```python
from build123d import *

# Parameters (mm, degrees)
SKETCH1_W           = 90
SKETCH1_H           = 34
BOSS_EXTRUDE1_DEPTH = 23.5
SKETCH2_R           = 1.8
BOSS_EXTRUDE4_DEPTH = 10
FILLET1_R           = 3


with BuildPart() as part:
    # Sketch1 → Boss-Extrude1 (new body)
    with BuildSketch(Plane(origin=(0, 0, 0), x_dir=(1, 0, 0), z_dir=(0, 1, 0))):
        with Locations((2.348643006, -1.686847599)):
            Rectangle(SKETCH1_W, SKETCH1_H)
    extrude(amount=BOSS_EXTRUDE1_DEPTH)

    # Sketch2 → Boss-Extrude4 (add)
    with BuildSketch(Plane(origin=(47.348643006, 0, 0), x_dir=(0, 0, -1), z_dir=(1, 0, 0))):
        with Locations(Location((-16.886847599, 13.57, 0), (0, 0, 180))):
            Circle(SKETCH2_R)
        with Locations(Location((-16.886847599, 9.93, 0), (0, 0, 180))):
            Circle(SKETCH2_R)
    extrude(amount=BOSS_EXTRUDE4_DEPTH)

    # Fillet1
    # the kernel refuses this fillet: 3 mm, written as the material it takes off along each edge
    with BuildSketch(Plane(origin=(44.348643006, 20.5, -12.313152401), x_dir=(1, 0, 0), z_dir=(0, 0, -1))) as fillet1_piece_1_section:
        Polygon((0, 0), (FILLET1_R * 1.02, 0), (FILLET1_R * 1.02, -FILLET1_R * 1.02), (0, -FILLET1_R * 1.02), align=None)
    fillet1_piece_1 = extrude(amount=FILLET1_R * 1.02, mode=Mode.PRIVATE)
    fillet1_piece_1 = fillet1_piece_1 - Plane(origin=(44.348643006, 20.5, -12.313152401), x_dir=(-0.7071067811865475, -0.7071067811865475, 0), z_dir=(0, 0, -1)) * Sphere(FILLET1_R, mode=Mode.PRIVATE)
    add(fillet1_piece_1, mode=Mode.SUBTRACT)
    with BuildSketch(Plane(origin=(44.348643006, 20.5, 15.686847599), x_dir=(0, 1, 0), z_dir=(1, 0, 0))) as fillet1_piece_2_section:
        Polygon((0, 0), (FILLET1_R * 1.02, 0), (FILLET1_R * 1.02, FILLET1_R * 1.02), (0, FILLET1_R * 1.02), align=None)
    fillet1_piece_2 = extrude(amount=FILLET1_R * 1.02, mode=Mode.PRIVATE)
    fillet1_piece_2 = fillet1_piece_2 - Plane(origin=(44.348643006, 20.5, 15.686847599), x_dir=(0, -0.7071067811865475, -0.7071067811865475), z_dir=(1, 0, 0)) * Sphere(FILLET1_R, mode=Mode.PRIVATE)
    add(fillet1_piece_2, mode=Mode.SUBTRACT)
    with BuildSketch(Plane(origin=(-39.651356994, 20.5, -12.313152401), x_dir=(-1, 0, 0), z_dir=(0, 0, -1))) as fillet1_piece_3_section:
        Polygon((0, 0), (FILLET1_R * 1.02, 0), (FILLET1_R * 1.02, FILLET1_R * 1.02), (0, FILLET1_R * 1.02), align=None)
    fillet1_piece_3 = extrude(amount=FILLET1_R * 1.02, mode=Mode.PRIVATE)
    fillet1_piece_3 = fillet1_piece_3 - Plane(origin=(-39.651356994, 20.5, -12.313152401), x_dir=(0.7071067811865475, -0.7071067811865475, 0), z_dir=(0, 0, -1)) * Sphere(FILLET1_R, mode=Mode.PRIVATE)
    add(fillet1_piece_3, mode=Mode.SUBTRACT)
    with BuildSketch(Plane(origin=(44.348643006, 3, 15.686847599), x_dir=(0, -1, 0), z_dir=(1, 0, 0))) as fillet1_piece_4_section:
        Polygon((0, 0), (FILLET1_R * 1.02, 0), (FILLET1_R * 1.02, -FILLET1_R * 1.02), (0, -FILLET1_R * 1.02), align=None)
    fillet1_piece_4 = extrude(amount=FILLET1_R * 1.02, mode=Mode.PRIVATE)
    fillet1_piece_4 = fillet1_piece_4 - Plane(origin=(44.348643006, 3, 15.686847599), x_dir=(0, 0.7071067811865475, -0.7071067811865475), z_dir=(1, 0, 0)) * Sphere(FILLET1_R, mode=Mode.PRIVATE)
    add(fillet1_piece_4, mode=Mode.SUBTRACT)
    with BuildSketch(Plane(origin=(-39.651356994, 20.5, 15.686847599), x_dir=(0, 1, 0), z_dir=(-1, 0, 0))) as fillet1_piece_5_section:
        Polygon((0, 0), (FILLET1_R * 1.02, 0), (FILLET1_R * 1.02, -FILLET1_R * 1.02), (0, -FILLET1_R * 1.02), align=None)
    fillet1_piece_5 = extrude(amount=FILLET1_R * 1.02, mode=Mode.PRIVATE)
    fillet1_piece_5 = fillet1_piece_5 - Plane(origin=(-39.651356994, 20.5, 15.686847599), x_dir=(0, -0.7071067811865475, -0.7071067811865475), z_dir=(-1, 0, 0)) * Sphere(FILLET1_R, mode=Mode.PRIVATE)
    add(fillet1_piece_5, mode=Mode.SUBTRACT)
    with BuildSketch(Plane(origin=(-39.651356994, 3, -12.313152401), x_dir=(-1, 0, 0), z_dir=(0, 0, -1))) as fillet1_piece_6_section:
        Polygon((0, 0), (FILLET1_R * 1.02, 0), (FILLET1_R * 1.02, -FILLET1_R * 1.02), (0, -FILLET1_R * 1.02), align=None)
    fillet1_piece_6 = extrude(amount=FILLET1_R * 1.02, mode=Mode.PRIVATE)
    fillet1_piece_6 = fillet1_piece_6 - Plane(origin=(-39.651356994, 3, -12.313152401), x_dir=(0.7071067811865475, 0.7071067811865475, 0), z_dir=(0, 0, -1)) * Sphere(FILLET1_R, mode=Mode.PRIVATE)
    add(fillet1_piece_6, mode=Mode.SUBTRACT)
    with BuildSketch(Plane(origin=(44.348643006, 3, -12.313152401), x_dir=(1, 0, 0), z_dir=(0, 0, -1))) as fillet1_piece_7_section:
        Polygon((0, 0), (FILLET1_R * 1.02, 0), (FILLET1_R * 1.02, FILLET1_R * 1.02), (0, FILLET1_R * 1.02), align=None)
    fillet1_piece_7 = extrude(amount=FILLET1_R * 1.02, mode=Mode.PRIVATE)
    fillet1_piece_7 = fillet1_piece_7 - Plane(origin=(44.348643006, 3, -12.313152401), x_dir=(-0.7071067811865475, 0.7071067811865475, 0), z_dir=(0, 0, -1)) * Sphere(FILLET1_R, mode=Mode.PRIVATE)
    add(fillet1_piece_7, mode=Mode.SUBTRACT)
    with BuildSketch(Plane(origin=(-39.651356994, 3, 15.686847599), x_dir=(0, -1, 0), z_dir=(-1, 0, 0))) as fillet1_piece_8_section:
        Polygon((0, 0), (FILLET1_R * 1.02, 0), (FILLET1_R * 1.02, FILLET1_R * 1.02), (0, FILLET1_R * 1.02), align=None)
    fillet1_piece_8 = extrude(amount=FILLET1_R * 1.02, mode=Mode.PRIVATE)
    fillet1_piece_8 = fillet1_piece_8 - Plane(origin=(-39.651356994, 3, 15.686847599), x_dir=(0, 0.7071067811865475, -0.7071067811865475), z_dir=(-1, 0, 0)) * Sphere(FILLET1_R, mode=Mode.PRIVATE)
    add(fillet1_piece_8, mode=Mode.SUBTRACT)
    with BuildSketch(Plane(origin=(47.348643006, 23.5, -12.313152401), x_dir=(0, -1, 0), z_dir=(0, 0, 1)), Plane(origin=(-42.651356994, 23.5, 15.686847599), x_dir=(0, -1, 0), z_dir=(0, 0, -1))) as fillet1_piece_9:
        with BuildLine():
            CenterArc((FILLET1_R, -FILLET1_R), FILLET1_R, 90, 90)
            Line((0, -FILLET1_R), (0, 0))
            Line((0, 0), (FILLET1_R, 0))
        make_face()
    extrude(amount=28, mode=Mode.SUBTRACT)
    with BuildSketch(Plane(origin=(-39.651356994, 23.5, -15.313152401), x_dir=(0, -1, 0), z_dir=(1, 0, 0)), Plane(origin=(44.348643006, 0, 18.686847599), x_dir=(0, 0, -1), z_dir=(-1, 0, 0))) as fillet1_piece_10:
        with BuildLine():
            CenterArc((FILLET1_R, -FILLET1_R), FILLET1_R, 90, 90)
            Line((0, -FILLET1_R), (0, 0))
            Line((0, 0), (FILLET1_R, 0))
        make_face()
    extrude(amount=84, mode=Mode.SUBTRACT)
    with BuildSketch(Plane(origin=(47.348643006, 9.93, 18.686847599), x_dir=(0, 0, -1), z_dir=(0, 1, 0))) as fillet1_piece_11_section:
        with BuildLine():
            CenterArc((FILLET1_R, FILLET1_R), FILLET1_R, 180, 90)
            Line((0, FILLET1_R), (0, 0))
            Line((0, 0), (FILLET1_R, 0))
        make_face()
    fillet1_piece_11 = extrude(amount=3.64, mode=Mode.PRIVATE)
    fillet1_piece_11 = fillet1_piece_11 - Plane(origin=(46.419832721, 13.57, 16.886847599), x_dir=(0, 0, 1), z_dir=(-1, 0, 0)) * Cylinder(1.8, 20, mode=Mode.PRIVATE)
    fillet1_piece_11 = fillet1_piece_11 - Plane(origin=(46.419832721, 9.93, 16.886847599), x_dir=(0, 0, 1), z_dir=(-1, 0, 0)) * Cylinder(1.8, 20, mode=Mode.PRIVATE)
    add(fillet1_piece_11, mode=Mode.SUBTRACT)
    with BuildSketch(Plane(origin=(47.348643006, 3, 18.686847599), x_dir=(0, 0, -1), z_dir=(0, 1, 0))) as fillet1_piece_12_section:
        with BuildLine():
            CenterArc((FILLET1_R, FILLET1_R), FILLET1_R, 180, 90)
            Line((0, FILLET1_R), (0, 0))
            Line((0, 0), (FILLET1_R, 0))
        make_face()
    fillet1_piece_12 = extrude(amount=6.93, mode=Mode.PRIVATE)
    fillet1_piece_12 = fillet1_piece_12 - Plane(origin=(46.65046867, 9.93, 16.886847599), x_dir=(0, 0, 1), z_dir=(-1, 0, 0)) * Cylinder(1.8, 26, mode=Mode.PRIVATE)
    add(fillet1_piece_12, mode=Mode.SUBTRACT)
    with BuildSketch(Plane(origin=(-39.651356994, 0, -15.313152401), x_dir=(0, 1, 0), z_dir=(1, 0, 0)), Plane(origin=(44.348643006, 23.5, 18.686847599), x_dir=(0, 0, -1), z_dir=(-1, 0, 0))) as fillet1_piece_13:
        with BuildLine():
            CenterArc((FILLET1_R, FILLET1_R), FILLET1_R, 180, 90)
            Line((0, FILLET1_R), (0, 0))
            Line((0, 0), (FILLET1_R, 0))
        make_face()
    extrude(amount=84, mode=Mode.SUBTRACT)
    with BuildSketch(Plane(origin=(47.348643006, 0, -12.313152401), x_dir=(0, 1, 0), z_dir=(0, 0, 1)), Plane(origin=(-42.651356994, 0, 15.686847599), x_dir=(0, 1, 0), z_dir=(0, 0, -1))) as fillet1_piece_14:
        with BuildLine():
            CenterArc((FILLET1_R, FILLET1_R), FILLET1_R, 180, 90)
            Line((0, FILLET1_R), (0, 0))
            Line((0, 0), (FILLET1_R, 0))
        make_face()
    extrude(amount=28, mode=Mode.SUBTRACT)
    with BuildSketch(Plane(origin=(-42.651356994, 3, -15.313152401), x_dir=(1, 0, 0), z_dir=(0, 1, 0)), Plane(origin=(-42.651356994, 3, 18.686847599), x_dir=(0, 0, -1), z_dir=(0, 1, 0))) as fillet1_piece_15:
        with BuildLine():
            CenterArc((FILLET1_R, -FILLET1_R), FILLET1_R, 90, 90)
            Line((0, -FILLET1_R), (0, 0))
            Line((0, 0), (FILLET1_R, 0))
        make_face()
    extrude(amount=17.5, mode=Mode.SUBTRACT)
    with BuildSketch(Plane(origin=(47.348643006, 3, -15.313152401), x_dir=(-1, 0, 0), z_dir=(0, 1, 0))) as fillet1_piece_16:
        with BuildLine():
            CenterArc((FILLET1_R, FILLET1_R), FILLET1_R, 180, 90)
            Line((0, FILLET1_R), (0, 0))
            Line((0, 0), (FILLET1_R, 0))
        make_face()
    extrude(amount=17.5, mode=Mode.SUBTRACT)
    with BuildSketch(Plane(origin=(47.348643006, 13.57, 18.686847599), x_dir=(0, 0, -1), z_dir=(0, 1, 0))) as fillet1_piece_17_section:
        with BuildLine():
            CenterArc((FILLET1_R, FILLET1_R), FILLET1_R, 180, 90)
            Line((0, FILLET1_R), (0, 0))
            Line((0, 0), (FILLET1_R, 0))
        make_face()
    fillet1_piece_17 = extrude(amount=6.93, mode=Mode.PRIVATE)
    fillet1_piece_17 = fillet1_piece_17 - Plane(origin=(46.65046859, 13.57, 16.886847599), x_dir=(0, 0, 1), z_dir=(-1, 0, 0)) * Cylinder(1.8, 26, mode=Mode.PRIVATE)
    add(fillet1_piece_17, mode=Mode.SUBTRACT)


solid = part.part
```
Verification items for the finished model (mm, model axes). Coordinates: 2 decimals unless noted, no trailing zeros. Write each loop counter-clockwise with the first axis right and the second up, starting at its lowest first coordinate (ties: lowest second). Pieces come first, ordered by that corner, then holes. Notation, with made-up numbers: M 76.5,55 L 91.5,55 A21 cw 91.5,91 Z; hole C -25.5,4.5 d7. An arc over 180 degrees is marked long. One line per item, written item: value.
Item 1: Gauge pin test, flat end, axial feed: pin 1 Ø8 at (y, z) = (19, 10) entering from +X. Record the tip position at first contact, or that the pin passes through.
Check sheet entries:
pin 1: stops at x = 47.35
Item 2: Section check A-A, the plane x = 50. Record the boundary of the cut face in (y, z), plus the area to 3 significant figures.
Check sheet entries:
outline: C 9.93,16.89 d3.6; C 13.57,16.89 d3.6
area: 20.4 mm^2
Item 3: Scan lines: line 1 along X through (y, z) = (9.75, 9); line 2 along Y through (x, z) = (-33, -12.5); line 3 along X through (y, z) = (15.75, 16). Record each from-to range of solid material in increasing order.
Check sheet entries:
line 1: x = -42.65 to 47.35
line 2: y = 0.01 to 23.49
line 3: x = -42.63 to 47.33
Item 4: Section check B-B, the plane z = 12. Record the boundary of the cut face in (x, y), plus the area to 3 significant figures.
Check sheet entries:
outline: M -42.65,3 A3 ccw -39.65,0 L 44.35,0 A3 ccw 47.35,3 L 47.35,20.5 A3 ccw 44.35,23.5 L -39.65,23.5 A3 ccw -42.65,20.5 Z
area: 2,110 mm^2
Item 5: Section check C-C, the plane y = 5.5. Record the boundary of the cut face in (x, z), plus the area to 3 significant figures.
Check sheet entries:
outline: M -42.65,-12.31 A3 ccw -39.65,-15.31 L 44.35,-15.31 A3 ccw 47.35,-12.31 L 47.35,15.69 A3 ccw 44.35,18.69 L -39.65,18.69 A3 ccw -42.65,15.69 Z
area: 3,050 mm^2
Item 6: Mould release check, pull along Y, two halves, no side actions. Record for faces 1 (the cylindrical face through (-41.8, 11.63, 17.78)), 2 (the cylindrical face through (46.45, 0.86, 1.49)), 3 (the flat face through (2, 23.5, 1)), 4 (the cylindrical face through (45.61, 11.74, 18.41)): pulls with the +Y half, pulls with the -Y half, needs draft (parallel to the pull), parting line crosses it, or undercut.
Check sheet entries:
face 1: needs draft
face 2: pulls with the -Y half
face 3: pulls with the +Y half
face 4: undercut
